Geometry check sheet. Reference: the model listing, model coordinates, mm. A direction names the side the tool comes from. Coordinates: 2 decimals unless noted, no trailing zeros. Write each loop counter-clockwise with the first axis right and the second up, starting at its lowest first coordinate (ties: lowest second). Pieces come first, ordered by that corner, then holes. Notation, with made-up numbers: M 2,58.5 L 49,58.5 A22 cw 49,90.5 Z; hole C 52.5,-37 d11. An arc over 180 degrees is marked long. Write item = value, one per line. Start each with the question number.
```python
from build123d import *

# Parameters (mm, degrees)
FILLET1_R           = 6
BOSS_EXTRUDE1_START = -19.5
SKETCH3_R           = 4.5
BOSS_EXTRUDE1_DEPTH = 12
BOSS_EXTRUDE1_TAPER = 5
FILLET2_R           = 6


with BuildPart() as part:
    # Sketch1 → Revolve1 (revolve)
    with BuildSketch(Plane.XY, mode=Mode.PRIVATE) as revolve1_sk:
        Polygon((0, 110), (-3, 110), (-3, 6), (-20, 6), (-20, 0), (0, 0), align=None)
    revolve(revolve1_sk.sketch.rotate(Axis((0, 110, 0), (0, -1, 0)), 270), axis=Axis((0, 110, 0), (0, -1, 0)))

    # Fillet1
    fillet1_edges = [part.edges().sort_by_distance(p)[0] for p in [
        (0, 6, -3),
    ]]
    fillet(fillet1_edges, radius=FILLET1_R)

    # Sketch2 → Revolve2 (revolve)
    with BuildSketch(Plane.XY, mode=Mode.PRIVATE) as revolve2_sk:
        with BuildLine():
            Line((-11.852035479, 98.544183465), (-13.266249042, 99.958397027))
            Line((-13.266249042, 99.958397027), (6.263312277, 121.648172237))
            ThreePointArc((6.263312277, 121.648172237), (9.466087356, 127.932074931), (16.432235768, 126.828454712))
            Line((16.432235768, 126.828454712), (-11.852035479, 98.544183465))
        make_face()
    revolve(revolve2_sk.sketch.rotate(Axis((-11.852035479, 98.544183465, 0), (0.7071067811865513, 0.7071067811865438, 0)), 180), axis=Axis((-11.852035479, 98.544183465, 0), (0.7071067811865513, 0.7071067811865438, 0)))

    # Sketch3 → Boss-Extrude1 (add)
    with BuildSketch(Plane(origin=(43.346073993, 43.346073993, 0), x_dir=(0, 0, 1), z_dir=(-0.7071067811865513, -0.7071067811865437, 0)).offset(BOSS_EXTRUDE1_START)):
        with Locations((0, 78.061915033)):
            Circle(SKETCH3_R)
    extrude(amount=BOSS_EXTRUDE1_DEPTH, taper=BOSS_EXTRUDE1_TAPER)

    # Fillet2
    fillet2_edges = [part.edges().sort_by_distance(p)[0] for p in [
        (0, 6, -20),
    ]]
    fillet(fillet2_edges, radius=FILLET2_R - 0.0001)  # a hair under: the kernel refuses the full size


solid = part.part
```
Q1. Draft check along X on faces 3 (the face through (-11.83, 98.52, -0.03)), 4 (the face through (-10.717, 102.787, -0.097)), 5 (the face through (3, 6, -9)). Enter one of: pulls with the +X half, pulls with the -X half, needs draft (parallel to the pull), parting line crosses it, or undercut.
Q2. Scan lines: L1, parallel to Y at x = 4, z = 2; L2, parallel to Y at x = -5.5, z = -2; L3, parallel to Y at x = 8, z = 1. Record each from-to range of solid material in increasing order.
Q3. Set-up check for faces 1 (the face through (-0.9, 59.03, 2.86)), 2 (the face through (0, 0, 0)): record each of +Z, -Z, +X, -X, +Y, -Y from which the full face is reachable in a straight line by a thin tool's end or side.
Q4. Gauge pin test, flat ends, axial feed: pin 1 (2 mm diameter, centred on x = -0.5, z = -13.5, fed in from +Y); pin 2 (22.5 mm diameter, centred on x = -1, z = 2.5, fed in from +Y); pin 3 (6 mm diameter, centred on x = -5, y = 75.5, fed in from -Z). Record the tip position at first contact, or that the pin passes through.
Q5. Cross-section at B-B on y = 14. Enter the section's corners in (x, z), and give its area (3 significant figures).
Values found:
q1.face_3 = pulls with the -X half
q1.face_4 = undercut
q1.face_5 = needs draft
q2.L1 = 0 to 8.06, 108.84 to 110.27, 111.13 to 118.13
q2.L2 = 0 to 6.89, 102.8 to 109.58
q2.L3 = 0 to 6.07, 113.94 to 126.76
q3.face_1 = none
q3.face_2 = +Z, -Z, +X, -X, -Y
q4.pin_1 = 6
q4.pin_2 = 128.18
q4.pin_3 = -2.24
q5.outline = C 0,0 d6
q5.area = 28.3 mm²
